The model under review builds one solid part; all positions refer to its coordinate system, in mm. A direction names the side the tool comes from. Coordinates: 2 decimals unless noted, no trailing zeros. Write each loop counter-clockwise with the first axis right and the second up, starting at its lowest first coordinate (ties: lowest second). Pieces come first, ordered by that corner, then holes. Notation, with made-up numbers: M 26,13.25 L 66,13.25 A27 ccw 66,42.25 Z; hole C -6.75,67 d3. An arc over 180 degrees is marked long. Answer as a JSON object with one key per item and string values.
```python
from build123d import *

# Parameters (mm, degrees)
BOSS_EXTRUDE3_DEPTH  = 3
SKETCH6_R            = 1.465
BOSS_EXTRUDE7_DEPTH  = 3
FILLET1_R            = 0.5
SKETCH7_R            = 2.9999999999999982
BOSS_EXTRUDE8_DEPTH  = 16.215
BOSS_EXTRUDE9_DEPTH  = 1.405
SKETCH9_R            = 2
CUT_EXTRUDE1_DEPTH   = 35
SKETCH10_R           = 1.5000000000000009
CUT_EXTRUDE2_DEPTH   = 35
CUT_EXTRUDE3_DEPTH   = 2.5
CUT_EXTRUDE4_START   = -2.5
SKETCH14_W           = 16.27
SKETCH14_H           = 3.999999999999999
CUT_EXTRUDE4_DEPTH   = 2.5
BOSS_EXTRUDE10_DEPTH = 0.59
BOSS_EXTRUDE11_DEPTH = 13.33
FILLET2_R            = 0.5
FILLET3_R            = 0.5
SKETCH12_R           = 1.5000000000000009
CUT_EXTRUDE5_DEPTH   = 0.5
FILLET4_R            = 0.5
CUT_EXTRUDE6_START   = -0.5
SKETCH17_R           = 1.5000000000000009
CUT_EXTRUDE6_DEPTH   = 0.5
FILLET5_R            = 0.5


with BuildPart() as part:
    # Sketch1 → Boss-Extrude3 (new, symmetric)
    with BuildSketch(Plane.XY):
        with BuildLine():
            ThreePointArc((2.9999999999999982, 2.9999999999999973), (2.1213203435596406, 0.8786796564403563), (-5.5e-16, 0))
            Line((0, 0), (36.5, 0))
            Line((36.5, 0), (36.5, 6))
            Line((36.5, 6), (19.23, 5.999999999999999))
            Line((19.23, 5.999999999999999), (15.480454164508112, 3.571071981637192))
            ThreePointArc((15.480454164508112, 3.571071981637192), (15.048841816271192, 3.4166611598413845), (14.593679363207029, 3.4710584241003293))
            Line((14.593679363207029, 3.4710584241003297), (7.67, 5.999999999999995))
            Line((7.67, 5.999999999999995), (0, 5.9999999999999964))
            ThreePointArc((1.8e-16, 5.9999999999999964), (2.1213203435596415, 5.121320343559639), (2.9999999999999982, 2.9999999999999982))
        make_face()
    extrude(amount=BOSS_EXTRUDE3_DEPTH, both=True)

    # Sketch6 → Boss-Extrude7 (add)
    with BuildSketch(Plane(origin=(36.5, 0, 0), x_dir=(0, 0, -1), z_dir=(1, 0, 0))):
        with Locations((0, 2.999999999999999)):
            Circle(SKETCH6_R)
    extrude(amount=BOSS_EXTRUDE7_DEPTH)

    # Fillet1
    fillet1_edges = [part.edges().sort_by_distance(p)[0] for p in [
        (39.5, 2.9999999999999987, 1.465),
    ]]
    fillet(fillet1_edges, radius=FILLET1_R)

    # Sketch7 → Boss-Extrude8 (add, symmetric)
    with BuildSketch(Plane.XY):
        with Locations((0, 2.9999999999999982)):
            Circle(SKETCH7_R)
    extrude(amount=BOSS_EXTRUDE8_DEPTH, both=True)

    # Sketch8 → Boss-Extrude9 (add, symmetric)
    with BuildSketch(Plane.XY):
        with BuildLine():
            Line((7.055802237198053, 5.999999999999995), (7.67, 5.999999999999995))
            Line((7.67, 5.999999999999995), (7.67, 2.7155970544612273))
            Line((7.67, 2.7155970544612273), (19.552760462470925, 2.7155970544612273))
            Line((19.552760462470925, 2.7155970544612273), (19.552760462470925, 5.999999999999999))
            Line((19.552760462470925, 5.999999999999999), (16.849844518078097, 9.600752353739953))
            ThreePointArc((16.849844518078097, 9.600752353739953), (14.873619928851438, 10.76977515573235), (12.649594170011149, 10.19899729819309))
            Line((12.649594170011149, 10.19899729819309), (7.055802237198053, 5.999999999999995))
        make_face()
    extrude(amount=BOSS_EXTRUDE9_DEPTH, both=True)

    # Sketch9 → Cut-Extrude1 (cut)
    with BuildSketch(Plane.XY.offset(16.215)):
        with Locations((0, 2.9999999999999982)):
            Circle(SKETCH9_R)
    extrude(amount=-CUT_EXTRUDE1_DEPTH, mode=Mode.SUBTRACT)

    # Sketch10 → Cut-Extrude2 (cut)
    with BuildSketch(Plane.XY.offset(1.405)):
        with Locations((14.450596871818059, 7.799749651933077)):
            Circle(SKETCH10_R)
    extrude(amount=-CUT_EXTRUDE2_DEPTH, mode=Mode.SUBTRACT)

    # Sketch11 → Cut-Extrude3 (cut)
    with BuildSketch(Plane.XY.offset(3)):
        with BuildLine():
            Line((20.021402411915382, 4.999999999999999), (35.5, 4.999999999999999))
            Line((35.5, 4.999999999999999), (35.5, 1))
            Line((35.5, 1), (4.265183612786801, 0.9999999999999961))
            Line((4.265183612786801, 0.9999999999999961), (3.4641016151377535, 1))
            ThreePointArc((3.4641016151377535, 1), (3.9999999999999982, 2.9999999999999982), (3.4641016151377535, 4.9999999999999964))
            Line((3.4641016151377535, 4.9999999999999964), (7.503517654742404, 4.9999999999999964))
            Line((7.503517654742404, 4.9999999999999964), (7.67, 4.9999999999999964))
            Line((7.67, 4.9999999999999964), (14.581839900445662, 2.475382903620951))
            ThreePointArc((14.581839900445662, 2.475382903620951), (15.035884938334876, 2.420860249555603), (15.46672588726192, 2.5741759140057563))
            Line((15.46672588726192, 2.5741759140057563), (19.23, 4.999999999999999))
            Line((19.23, 4.999999999999999), (20.021402411915382, 4.999999999999999))
        make_face()
    extrude(amount=-CUT_EXTRUDE3_DEPTH, mode=Mode.SUBTRACT)

    # Sketch14 → Cut-Extrude4 (cut)
    with BuildSketch(Plane(origin=(0, 0, -3), x_dir=(-1, 0, 0), z_dir=(0, 0, -1)).offset(CUT_EXTRUDE4_START)):
        with BuildLine():
            Line((-15.480454164508119, 2.571071981637197), (-19.23, 4.999999999999999))
            Line((-19.23, 4.999999999999999), (-19.23, 1))
            Line((-19.23, 1), (-3.5413002095084885, 1))
            Line((-3.5413002095084876, 1), (-3.4641016151377535, 1))
            ThreePointArc((-3.4641016151377535, 1), (-3.999999999999998, 2.9999999999999982), (-3.4641016151377535, 4.9999999999999964))
            Line((-3.4641016151377535, 4.9999999999999964), (-7.67, 4.9999999999999964))
            Line((-7.67, 4.9999999999999964), (-14.593679363207022, 2.471058424100332))
            ThreePointArc((-14.593679363207022, 2.471058424100332), (-15.048841816271192, 2.4166611598413854), (-15.480454164508119, 2.5710719816371976))
        make_face()
        with Locations((-27.365000000000002, 2.9999999999999996)):
            Rectangle(SKETCH14_W, SKETCH14_H)
    extrude(amount=CUT_EXTRUDE4_DEPTH, mode=Mode.SUBTRACT)

    # Sketch15 → Boss-Extrude10 (add, symmetric)
    with BuildSketch(Plane.XY):
        with BuildLine():
            Line((11.889999999999997, -3.01e-15), (11.889999999999997, -3.750000000000003))
            Line((11.889999999999997, -3.750000000000003), (9.987882758608185, -5.652117241391816))
            Line((9.987882758608185, -5.652117241391816), (0.9878827586081856, -5.652117241391818))
            Line((0.9878827586081856, -5.652117241391818), (-2.7244278426211888, -1.9398066401624436))
            Line((-2.7244278426211888, -1.9398066401624436), (-2.7244278426211888, 1.7440171456781548))
            ThreePointArc((-2.7244278426211888, 1.7440171456781548), (-1.6174132800608587, 0.47334721786258305), (0, 0))
            Line((0, 0), (11.889999999999997, -3.01e-15))
        make_face()
    extrude(amount=BOSS_EXTRUDE10_DEPTH, both=True)

    # Sketch16 → Boss-Extrude11 (add, symmetric)
    with BuildSketch(Plane.XY):
        with BuildLine():
            Line((3.9580398915498063, 2.4999999999999982), (3.9580398915498063, 3.4999999999999982))
            Line((3.9580398915498063, 3.4999999999999982), (2.9580398915498067, 3.4999999999999982))
            ThreePointArc((2.9580398915498067, 3.4999999999999982), (2.9999999999999925, 2.9999999999999982), (2.9580398915498067, 2.4999999999999982))
            Line((2.9580398915498067, 2.4999999999999982), (3.9580398915498063, 2.4999999999999982))
        make_face()
    extrude(amount=BOSS_EXTRUDE11_DEPTH, both=True)

    # Fillet2
    fillet2_edges = [part.edges().sort_by_distance(p)[0] for p in [
        (3.9580398915498063, 2.9999999999999982, 13.33),
    ]]
    fillet(fillet2_edges, radius=FILLET2_R)

    # Fillet3
    fillet3_edges = [part.edges().sort_by_distance(p)[0] for p in [
        (3.9580398915498063, 2.9999999999999982, -13.33),
    ]]
    fillet(fillet3_edges, radius=FILLET3_R)

    # Sketch12 → Cut-Extrude5 (cut)
    with BuildSketch(Plane.XY.offset(1.405)):
        with BuildLine():
            Line((8.93667028661393, 5.537336294370084), (11.950596871818057, 7.799749651933077))
            ThreePointArc((11.950596871818057, 7.799749651933077), (14.45059687181806, 5.299749651933041), (16.950596871818053, 7.7997496519330864))
            Line((16.95059687181806, 7.799749651933077), (18.60533758587746, 5.595348315169656))
            Line((18.60533758587746, 5.595348315169656), (19.230000000000004, 5.999999999999997))
            Line((19.230000000000004, 5.999999999999997), (19.552760462470925, 5.999999999999999))
            Line((19.552760462470925, 5.999999999999999), (16.849844518078097, 9.600752353739953))
            ThreePointArc((16.849844518078097, 9.600752353739953), (14.873619928851436, 10.769775155732342), (12.649594170011149, 10.19899729819309))
            Line((12.649594170011149, 10.19899729819309), (7.055802237198053, 5.999999999999995))
            Line((7.055802237198053, 5.999999999999995), (7.67, 5.999999999999995))
            Line((7.67, 5.999999999999995), (8.93667028661393, 5.537336294370084))
        make_face()
        with Locations((14.450596871818059, 7.799749651933077)):
            Circle(SKETCH12_R, mode=Mode.SUBTRACT)
    extrude(amount=-CUT_EXTRUDE5_DEPTH, mode=Mode.SUBTRACT)

    # Fillet4
    fillet4_edges = [part.edges().sort_by_distance(p)[0] for p in [
        (18.20130249027451, 7.800376176869976, 0.905),
        (9.8526982036046, 8.099498649096542, 0.905),
        (14.873619928851436, 10.769775155732344, 0.905),
    ]]
    fillet(fillet4_edges, radius=FILLET4_R)

    # Sketch17 → Cut-Extrude6 (cut)
    with BuildSketch(Plane(origin=(0, 0, -1.405), x_dir=(-1, 0, 0), z_dir=(0, 0, -1)).offset(CUT_EXTRUDE6_START)):
        with BuildLine():
            Line((-18.60533758587746, 5.595348315169656), (-16.95059687181806, 7.799749651933077))
            ThreePointArc((-16.95059687181806, 7.799749651933077), (-14.450596871818068, 5.299749651933066), (-11.950596871818057, 7.79974965193306))
            Line((-11.950596871818059, 7.799749651933077), (-8.93667028661393, 5.537336294370084))
            Line((-8.93667028661393, 5.537336294370084), (-7.67, 5.999999999999995))
            Line((-7.67, 5.999999999999995), (-7.055802237198053, 5.999999999999995))
            Line((-7.055802237198053, 5.999999999999995), (-12.649594170011149, 10.19899729819309))
            ThreePointArc((-12.649594170011149, 10.19899729819309), (-14.873619928851438, 10.769775155732347), (-16.849844518078097, 9.600752353739953))
            Line((-16.849844518078097, 9.600752353739953), (-19.552760462470925, 5.999999999999999))
            Line((-19.552760462470925, 5.999999999999999), (-19.23, 5.999999999999999))
            Line((-19.23, 5.999999999999999), (-18.60533758587746, 5.595348315169656))
        make_face()
        with Locations(Location((-14.450596871818059, 7.799749651933077, 0), (0, 0, 180))):
            Circle(SKETCH17_R, mode=Mode.SUBTRACT)
    extrude(amount=CUT_EXTRUDE6_DEPTH, mode=Mode.SUBTRACT)

    # Fillet5
    fillet5_edges = [part.edges().sort_by_distance(p)[0] for p in [
        (9.8526982036046, 8.099498649096542, -0.905),
        (18.20130249027451, 7.800376176869976, -0.905),
        (14.873619928851438, 10.769775155732347, -0.905),
    ]]
    fillet(fillet5_edges, radius=FILLET5_R)


solid = part.part
```
(1) Add section B-B on z = 6.5. Give the boundary of the cut face in (x, y), and give its area (3 significant figures).
Results list:
{"outline": "M 2.96,2.5 L 3.96,2.5 L 3.96,3.5 L 2.96,3.5 A3 ccw long Z; hole C 0,3 d4", "area": "16.7 mm²"}
(2) Add section C-C on x = 33. Give the boundary of the cut face in (y, z), and give its area (3 significant figures).
Results list:
{"outline": "M 0,-3 L 1,-3 L 1,-0.5 L 5,-0.5 L 5,-3 L 6,-3 L 6,3 L 5,3 L 5,0.5 L 1,0.5 L 1,3 L 0,3 Z", "area": "16.0 mm²"}
(3) For faces 1 (the face through (3.5, 3.5, 8.2)), 2 (the face through (-2.724, 0, 0)), 3 (the face through (-2.21, 5.03, 0.23)), 4 (the face through (10.46, 6.68, -1.15)), 5 (the face through (27, 5, -2)), list the 3-axis set-ups (+Z, -Z, +X, -X, +Y, -Y) from which the entire face can be reached by the end or side of a thin tool; tool diameter is ignored.
Results list:
{"face 1": "+Z, +X, +Y", "face 2": "+Z, -Z, -X, -Y", "face 3": "none", "face 4": "-Z, +Y", "face 5": "-Z"}
(4) Add section A-A on x = 6. Give the boundary of the cut face in (y, z), and give its area (3 significant figures).
Results list:
{"outline": "M -5.65,-0.59 L 0,-0.59 L 0,-3 L 1,-3 L 1,-0.5 L 5,-0.5 L 5,-3 L 6,-3 L 6,3 L 5,3 L 5,0.5 L 1,0.5 L 1,3 L 0,3 L 0,0.59 L -5.65,0.59 Z", "area": "22.7 mm²"}
(5) Draft analysis for pull direction X (two halves, no side actions). For faces 6 (the face through (20.9, 0.8, 3)), 7 (the face through (20, 3, -0.5)), 8 (the face through (-0.842, -3.822, 0.008)), state which applies: released by +X, released by -X, zero draft, split by the parting line, or undercut.
Results list:
{"face 6": "zero draft", "face 7": "undercut", "face 8": "released by -X"}
(6) Wall thickness on line 1 along Y through (x, z) = (0, -7); line 2 along X through (y, z) = (2.25, -1); line 3 along Z through (x, y) = (23, 0.75): over which ranges is each line inside the solid? List them lowest first. Write a range as from..to.
Results list:
{"line 1": "0..1, 5..6", "line 2": "-2.9..-1.85, 1.85..3.93, 35.5..39.41", "line 3": "-3..3"}
(7) For pin 1 Ø6 at (x, y) = (14, 0) entering from -Z; pin 2 Ø0.5 at (x, z) = (3.5, -10) entering from +Y; pin 3 Ø4 at (y, z) = (-3.5, 6) entering from -X; pin 4 Ø0.8 at (x, z) = (3.5, 10) entering from -Y, all flat-tipped, find the tip position at first contact; note any pin that passes through.
Results list:
{"pin 1": "z = -3", "pin 2": "y = 3.5", "pin 3": "through", "pin 4": "y = 2.5"}
